Check sheet for the modelled part. Datum: model origin and axes. Units: mm. Round coordinates to 2 decimals unless told otherwise and drop trailing zeros. Order: outer loops, then holes, each group sorted by start corner. A loop starts at its lowest first (then second) coordinate and runs counter-clockwise, first axis right, second up.
Q1. Cross-section at D-D on z = -70. Record the cut outline in (x, y) (3 decimals), then the cut area to 3 significant figures.
Q2. Cross-section at C-C on x = -73. Record the cut outline in (y, z) (3 decimals).
Q3. Cross-section at A-A on y = -2.5. Give the number of separate pieces and of enclosed holes in the cut face, then the cut area to 3 significant figures.
Q4. Cross-section at B-B on z = -109. Record the cut outline in (x, y) (3 decimals).
Q5. Mould release check, pull along X, two halves, no side actions. Record for faces 1 (the flat face through (-12, -6.35, 23)), 2 (the cylindrical face through (-57.758, -3.131, -58.979)), 3 (the cylindrical face through (-118.42, -3.13, -90.8)): +X half, -X half, draft (parallel to the pull), parting line (faces both ways), or undercut.
Q6. Depth check by flat-ended pin: P1, Ø1.9, axis at y = -2, z = -112, coming from the +X side; P2, Ø1, axis at x = 55.5, y = -4, coming from the +Z side; P3, Ø1.5, axis at x = -44.5, z = -73.5, coming from the +Y side; P4, Ø1.9, axis at x = -68, y = -4.5, coming from the +Z side. Enter the tip coordinate at first touch or a pass-through.
Q7. Scan lines: probe 1 along X at (y, z) = (-0.75, 50) (3 decimals); probe 2 along X at (y, z) = (-4, -68) (3 decimals); probe 3 along Z at (x, y) = (-36, -3.75) (3 decimals). Record each from-to range of solid material in increasing order.
from build123d import *

# Parameters (mm, degrees)
F0_R     = 149.225
F0_R_2   = 25.399996
F1_DEPTH = 6.35


with BuildPart() as f1:
    # F0 (on Front) → F1 (new body)
    with BuildSketch(Plane.XZ):
        Circle(F0_R)
        with BuildLine():
            ThreePointArc((-3.175, -139.663916), (-98.782817, -98.782817), (-139.663916, -3.175))
            Line((-139.663916, -3.175), (-88.843285, -3.175))
            ThreePointArc((-88.843285, -3.175), (-62.861793, -62.861793), (-3.175, -88.843285))
            Line((-3.175, -88.843285), (-3.175, -139.663916))
        make_face(mode=Mode.SUBTRACT)
        with BuildLine():
            ThreePointArc((-3.175, -82.488916), (-58.371662, -58.371662), (-82.488916, -3.175))
            Line((-82.488916, -3.175), (-31.590848, -3.175))
            ThreePointArc((-31.590848, -3.175), (-22.450638, -22.450638), (-3.175, -31.590848))
            Line((-3.175, -31.590848), (-3.175, -82.488916))
        make_face(mode=Mode.SUBTRACT)
        with BuildLine():
            Line((3.175, -139.663916), (3.175, -88.843285))
            ThreePointArc((3.175, -88.843285), (62.861793, -62.861793), (88.843285, -3.175))
            Line((88.843285, -3.175), (139.663916, -3.175))
            ThreePointArc((139.663916, -3.175), (98.782817, -98.782817), (3.175, -139.663916))
        make_face(mode=Mode.SUBTRACT)
        with BuildLine():
            Line((3.175, -82.488916), (3.175, -31.590848))
            ThreePointArc((3.175, -31.590848), (22.450638, -22.450638), (31.590848, -3.175))
            Line((31.590848, -3.175), (31.749997, -3.175))
            Line((31.749997, -3.175), (82.488916, -3.175))
            ThreePointArc((82.488916, -3.175), (58.371662, -58.371662), (3.175, -82.488916))
        make_face(mode=Mode.SUBTRACT)
        with BuildLine():
            Line((-31.590848, 3.175), (-31.749997, 3.175))
            Line((-31.749997, 3.175), (-82.488916, 3.175))
            ThreePointArc((-82.488916, 3.175), (-58.371662, 58.371662), (-3.175, 82.488916))
            Line((-3.175, 82.488916), (-3.175, 31.749997))
            Line((-3.175, 31.749997), (-3.175, 31.590848))
            ThreePointArc((-3.175, 31.590848), (-22.450638, 22.450638), (-31.590848, 3.175))
        make_face(mode=Mode.SUBTRACT)
        with BuildLine():
            ThreePointArc((-139.663916, 3.175), (-98.782817, 98.782817), (-3.175, 139.663916))
            Line((-3.175, 139.663916), (-3.175, 88.843285))
            ThreePointArc((-3.175, 88.843285), (-62.861793, 62.861793), (-88.843285, 3.175))
            Line((-88.843285, 3.175), (-139.663916, 3.175))
        make_face(mode=Mode.SUBTRACT)
        Circle(F0_R_2, mode=Mode.SUBTRACT)
        with BuildLine():
            Line((3.175, 31.590848), (3.175, 31.749997))
            Line((3.175, 31.749997), (3.175, 82.488916))
            ThreePointArc((3.175, 82.488916), (58.371662, 58.371662), (82.488916, 3.175))
            Line((82.488916, 3.175), (31.590848, 3.175))
            ThreePointArc((31.590848, 3.175), (22.450638, 22.450638), (3.175, 31.590848))
        make_face(mode=Mode.SUBTRACT)
        with BuildLine():
            ThreePointArc((3.175, 139.663916), (98.782817, 98.782817), (139.663916, 3.175))
            Line((139.663916, 3.175), (88.843285, 3.175))
            ThreePointArc((88.843285, 3.175), (62.861793, 62.861793), (3.175, 88.843285))
            Line((3.175, 88.843285), (3.175, 139.663916))
        make_face(mode=Mode.SUBTRACT)
    extrude(amount=F1_DEPTH)


solid = f1.part
Results found:
1. outline: (-131.788, -6.35) - (-120.897, -6.35) - (-120.897, 0) - (-131.788, 0) - close; (-54.802, -6.35) - (-43.755, -6.35) - (-43.755, 0) - (-54.802, 0) - close; (-3.175, -6.35) - (3.175, -6.35) - (3.175, 0) - (-3.175, 0) - close; (43.755, -6.35) - (54.802, -6.35) - (54.802, 0) - (43.755, 0) - close; (120.897, -6.35) - (131.788, -6.35) - (131.788, 0) - (120.897, 0) - close
1. area: 319 mm2
2. outline: (-6.35, -130.15) - (0, -130.15) - (0, -119.11) - (-6.35, -119.11) - close; (-6.35, -50.737) - (0, -50.737) - (0, -38.542) - (-6.35, -38.542) - close; (-6.35, -3.175) - (0, -3.175) - (0, 3.175) - (-6.35, 3.175) - close; (-6.35, 38.542) - (0, 38.542) - (0, 50.737) - (-6.35, 50.737) - close; (-6.35, 119.11) - (0, 119.11) - (0, 130.15) - (-6.35, 130.15) - close
3. separate pieces: 1
3. enclosed holes: 9
3. area: 15,800 mm2
4. outline: (-101.917, -6.35) - (-87.379, -6.35) - (-87.379, 0) - (-101.917, 0) - close; (-3.175, -6.35) - (3.175, -6.35) - (3.175, 0) - (-3.175, 0) - close; (87.379, -6.35) - (101.917, -6.35) - (101.917, 0) - (87.379, 0) - close
5. face 1: draft
5. face 2: undercut
5. face 3: parting line
6. P1: stops at x = 99.68
6. P2: stops at z = 138.72
6. P3: stops at y = 0
6. P4: stops at z = 133.31
7. probe 1: x = -140.599 to -130.446, -73.507 to -65.685, -3.175 to 3.175, 65.685 to 73.507, 130.446 to 140.599
7. probe 2: x = -132.831 to -122.033, -57.264 to -46.803, -3.175 to 3.175, 46.803 to 57.264, 122.033 to 132.831
7. probe 3: z = -144.817 to -134.982, -81.285 to -74.287, -3.175 to 3.175, 74.287 to 81.285, 134.982 to 144.817
